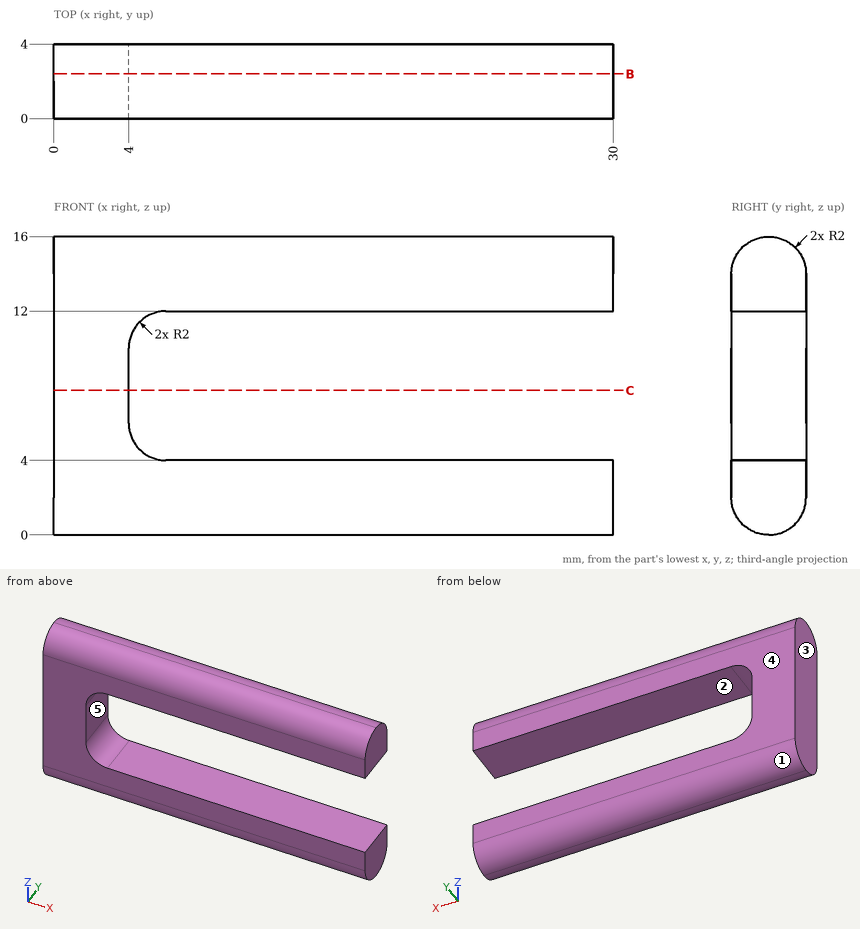
Check sheet for the drawn part. Datum: minimum x, y, z corner. Units: mm. A direction names the side the tool comes from. Round coordinates to 2 decimals unless told otherwise and drop trailing zeros. Write each loop counter-clockwise with the first axis right and the second up, starting at its lowest first coordinate (ties: lowest second). Pieces come first, ordered by that corner, then holes. Notation, with made-up numbers: (2, -30.75) -> (50, -30.75) arc R37 ccw to (50, 7.25) -> close; hole circle Ø9 at (-22.75, -27). An arc over 180 degrees is marked (long way). One line per item, written item: value. Start each with the question number.
(1) Cross-section at C-C, the plane z = 7.75. Record the cut outline in (x, y), and give its area (3 significant figures).
(2) Draft check along Z on the marked faces 1, 2 and 3. Enter one of: +Z half, -Z half, draft (parallel to the pull), parting line (faces both ways), or undercut.
(3) Cross-section at B-B, the plane y = 2.4. Record the cut outline in (x, z).
(4) Scan lines: line 1 (Z direction, x = 16.5, y = 1.95); line 2 (X direction, y = 1.4, z = 6.5); line 3 (Z direction, x = 6.5, y = 0.2). Record each from-to range of solid material in increasing order. Write a range as [from, to].
(5) Access from +Z, -Z, +X, -X, +Y, -Y to the whole of each face (thin tool, end or side, straight path). Record for the marked faces 4 and 5.
Answer:
1. outline: (0, 0) -> (4, 0) -> (4, 4) -> (0, 4) -> close
1. area: 16.0 mm²
2. face 1: -Z half
2. face 2: undercut
2. face 3: draft
3. outline: (0, 0.04) -> (30, 0.04) -> (30, 4) -> (6, 4) arc R2 cw to (4, 6) -> (4, 10) arc R2 cw to (6, 12) -> (30, 12) -> (30, 15.96) -> (0, 15.96) -> close
4. line 1: [0, 4], [12, 16]
4. line 2: [0, 4]
4. line 3: [1.13, 4], [12, 14.87]
5. face 4: +Z, -Z, +X, -X, +Y
5. face 5: +X, +Y, -Y
